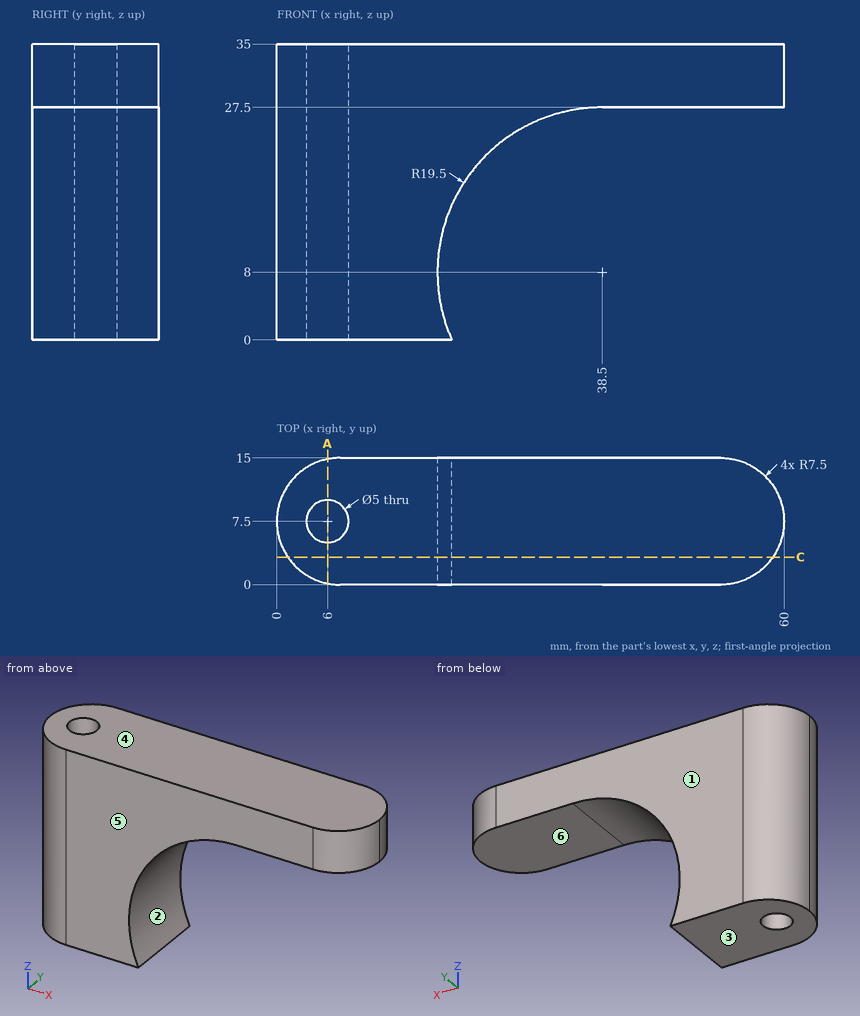
The figure shows three views and two pictorial views of one solid part (mm, origin at its lowest corner). Answer the questions. A direction names the side the tool comes from. Round coordinates to 2 decimals unless told otherwise and drop trailing zeros. Write each loop counter-clockwise with the first axis right and the second up, starting at its lowest first coordinate (ties: lowest second). Pieces come first, ordered by that corner, then holes. Notation, with made-up numbers: (88.25, 43) - (101.25, 43) arc R16 ccw to (101.25, 70) - close; hole circle Ø4 at (76, 82.25). An arc over 180 degrees is marked (long way). Use one line per item in the form item = value. Start each with the question number.
Item 1: Find the intervals of material crossed by line 1 (Y direction, x = 6, z = 18); line 2 (X direction, y = 7.25, z = 10); line 3 (Z direction, x = 40, y = 11), in increasing order. Write a range as [from, to].
Item 2: Determine the mould class of the marked faces 1, 2, 3 and 4 for opening direction Z: +Z half, -Z half, draft (parallel to the pull), parting line (faces both ways), or undercut.
Item 3: A tool of negligible diameter and unlimited length cuts with its end or side. For the marked faces 5 and 6, from which of +Z, -Z, +X, -X, +Y, -Y can it reach the whole face along a straight path? Write none if from no direction.
Item 4: Flat-ended cylindrical pins translate along their axes: pin 1 Ø3 at (x, z) = (7, 22) entering from +Y; pin 2 Ø6 at (x, y) = (37.5, 6.5) entering from -Z; pin 3 Ø3 at (y, z) = (12, 10.5) entering from +X; pin 4 Ø3 at (y, z) = (12, 20) entering from +X. Find the tip coordinate at first contact, or state that the pin passes through.
Item 5: A cutting plane is placed at C-C (y = 3.25). Write down the section's boundary in (x, z).
Item 6: A cutting plane is placed at A-A (x = 6). Write down the section's boundary in (y, z), plus the area to 3 significant figures.
The answers:
q1.line_1 = [0.15, 5], [10, 14.85]
q1.line_2 = [0, 3.51], [8.49, 19.1]
q1.line_3 = [27.5, 35]
q2.face_1 = draft
q2.face_2 = undercut
q2.face_3 = -Z half
q2.face_4 = +Z half
q3.face_5 = +Z, -Z, +X, -X, -Y
q3.face_6 = -Z, +X, +Y, -Y
q4.pin_1 = 15
q4.pin_2 = 27.09
q4.pin_3 = 19.41
q4.pin_4 = 24.43
q5.outline = (1.32, 0) - (20.72, 0) arc R19.5 cw to (38.5, 27.5) - (58.68, 27.5) - (58.68, 35) - (1.32, 35) - close
q6.outline = (0.15, 0) - (5, 0) - (5, 35) - (0.15, 35) - close; (10, 0) - (14.85, 0) - (14.85, 35) - (10, 35) - close
q6.area = 339 mm^2
